Input: dimensioned drawing with shaded views. Units: mm. Origin: part minimum x, y, z. Coordinates: 2 decimals unless noted, no trailing zeros. Loops run counter-clockwise (first coordinate to the right, second up) from the corner with the lowest first, then second, coordinate; pieces in that order, holes last.
Item 1: Section A-A on x = 273.5. Return loops of the section in (y, z).
Item 2: Contact query for flat-ended pins moving along their axis: P1, Ø6, axis at y = 4, z = 470, coming from the -X side; P2, Ø2, axis at y = 2.5, z = 302.5, coming from the +X side; P3, Ø6, axis at y = 8.5, z = 346, coming from the -X side; P4, Ø4, axis at x = 493.5, y = 6.5, coming from the -Z side. Output: stop coordinate, or through.
Item 3: Section B-B on z = 134.5. Return loops of the section in (x, y), and give its area (3 significant figures).
Item 4: Section D-D on x = 452. Return loops of the section in (y, z).
Item 5: Ray query, line 1 along Z through (x, y) = (523.5, 9.75); line 2 along X through (y, z) = (10.5, 136); line 3 along Z through (x, y) = (34.5, 7.5). Return the intervals inside material, ascending.
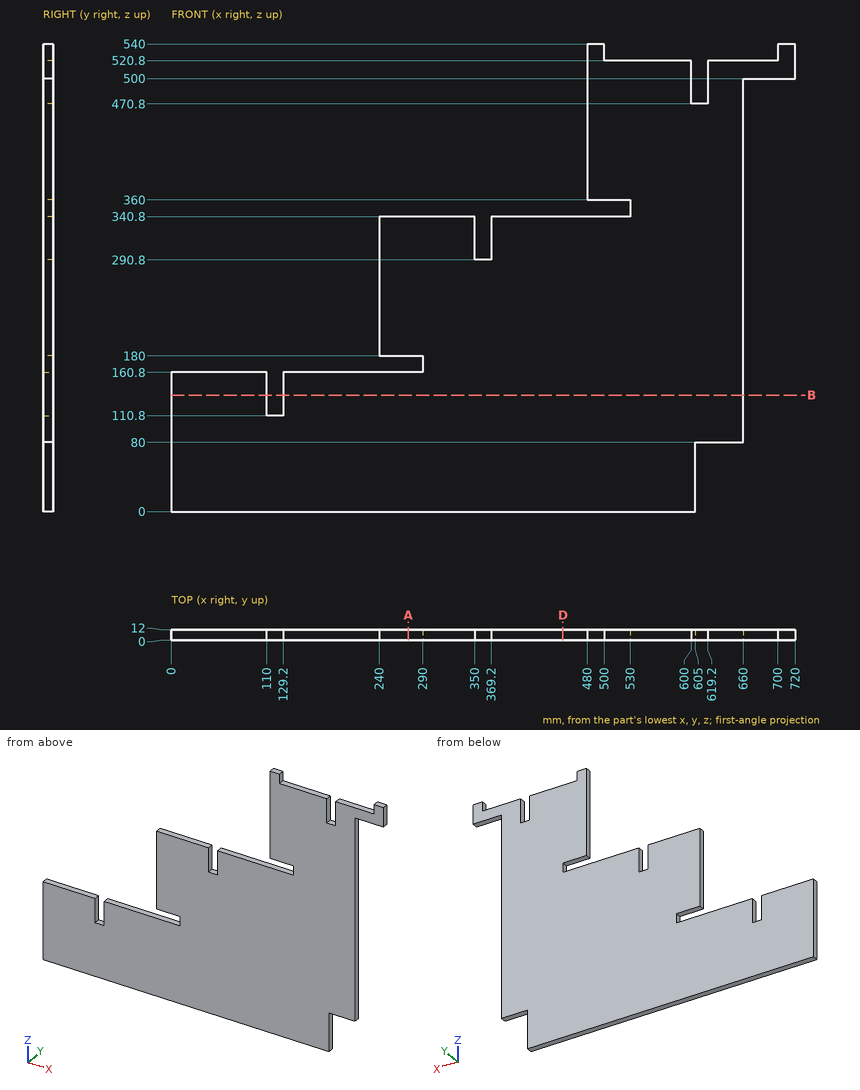
Results found:
1. outline: (0, 0) - (12, 0) - (12, 160.8) - (0, 160.8) - close; (0, 180) - (12, 180) - (12, 340.8) - (0, 340.8) - close
2. P1: stops at x = 480
2. P2: stops at x = 660
2. P3: stops at x = 530
2. P4: stops at z = 0
3. outline: (0, 0) - (110, 0) - (110, 12) - (0, 12) - close; (129.2, 0) - (660, 0) - (660, 12) - (129.2, 12) - close
3. area: 7,690 mm2
4. outline: (0, 0) - (12, 0) - (12, 340.8) - (0, 340.8) - close
5. line 1: z = 0 to 340.8, 360 to 520.8
5. line 2: x = 0 to 110, 129.2 to 660
5. line 3: z = 0 to 160.8
